The model under review builds one solid part; all positions refer to its coordinate system, in mm. Face numbers are marked on the shaded views. A direction names the side the tool comes from. Round coordinates to 2 decimals unless told otherwise and drop trailing zeros. Order: outer loops, then holes, each group sorted by start corner. A loop starts at its lowest first (then second) coordinate and runs counter-clockwise, first axis right, second up. Notation, with made-up numbers: M 74.25,32.25 L 88.25,32.25 A13 cw 88.25,42.25 Z; hole C 70,-8 d3. An arc over 180 degrees is marked long. Answer as CSV lines item,"result". Start each with the question number.
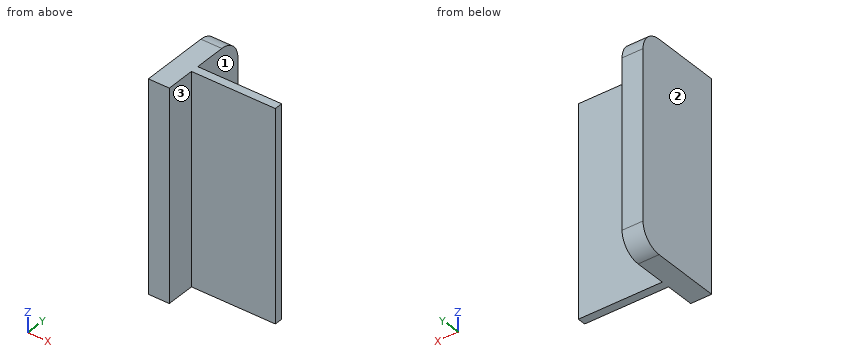
from build123d import *

# Parameters (mm, degrees)
F0_W     = 25.4
F0_H     = 50.8
F1_DEPTH = 2
F2_W     = 5.08
F2_H     = 50.8
F3_DEPTH = 7
F4_W     = 5.08
F4_H     = 50.8
F5_DEPTH = 12.7
F6_R     = 5.08


with BuildPart() as f1:
    # F0 (on Front) → F1 (new body)
    with BuildSketch(Plane.XZ):
        with Locations((12.7, 25.4)):
            Rectangle(F0_W, F0_H)
    extrude(amount=F1_DEPTH)

    # F2 (on face) → F3 (join)
    with BuildSketch(Plane.XZ.offset(2)):
        with Locations((2.54, 25.4)):
            Rectangle(F2_W, F2_H)
    extrude(amount=F3_DEPTH)

    # F4 (on face) → F5 (join)
    with BuildSketch(Plane(origin=(0, 0, 0), x_dir=(-1, 0, 0), z_dir=(0, 1, 0))):
        with Locations((-2.54, 25.4)):
            Rectangle(F4_W, F4_H)
    extrude(amount=F5_DEPTH)

    # F6
    f6_edges = [f1.edges().sort_by_distance(p)[0] for p in [
        (2.54, 12.7, 50.8),
        (2.54, 12.7, 0),
    ]]
    fillet(f6_edges, radius=F6_R)


solid = f1.part
Item 1: Wall thickness on probe 1 along Y at (x, z) = (24.75, 11); probe 2 along X at (y, z) = (2, 22): over which ranges is each line inside the solid? List them lowest first. Write a range as [from, to].
Item 2: Consider section B-B (y = 3.25). State the section outline as (x, z) points, and give its area (3 significant figures).
Item 3: Consider section A-A (z = 20). State the section outline as (x, y) points, and give its area (3 significant figures).
Item 4: Tool access review of the marked faces 1, 2 and 3: name each direction out of +Z, -Z, +X, -X, +Y, -Y from which nothing blocks a thin tool from reaching the whole face with its end or side.
Item 5: For pin 1 (5 mm diameter, centred on y = 8.5, z = 20, fed in from +X); pin 2 (5 mm diameter, centred on x = 10.5, z = 31, fed in from +Y); pin 3 (1 mm diameter, centred on x = 7, z = 14, fed in from -Y), all flat-tipped, find the tip position at first contact; note any pin that passes through.
Item 6: Consider section C-C (x = 12.75). State the section outline as (y, z) points.
Item 7: Consider section D-D (z = 47). State the section outline as (x, y) points.
Reported:
1,probe 1,"y = [-2, 0]"
1,probe 2,"x = [0, 5.08]"
2,outline,"M 0,0 L 5.08,0 L 5.08,50.8 L 0,50.8 Z"
2,area,"258 mm²"
3,outline,"M 0,-9 L 5.08,-9 L 5.08,-2 L 25.4,-2 L 25.4,0 L 5.08,0 L 5.08,12.7 L 0,12.7 Z"
3,area,"151 mm²"
4,face 1,"+Z, -Z, +X, +Y"
4,face 2,"+Z, -Z, -X, +Y, -Y"
4,face 3,"+Z, -Z, +X, -Y"
5,pin 1,"stops at x = 5.08"
5,pin 2,"stops at y = 0"
5,pin 3,"stops at y = -2"
6,outline,"M -2,0 L 0,0 L 0,50.8 L -2,50.8 Z"
7,outline,"M 0,-9 L 5.08,-9 L 5.08,-2 L 25.4,-2 L 25.4,0 L 5.08,0 L 5.08,12.54 L 0,12.54 Z"
